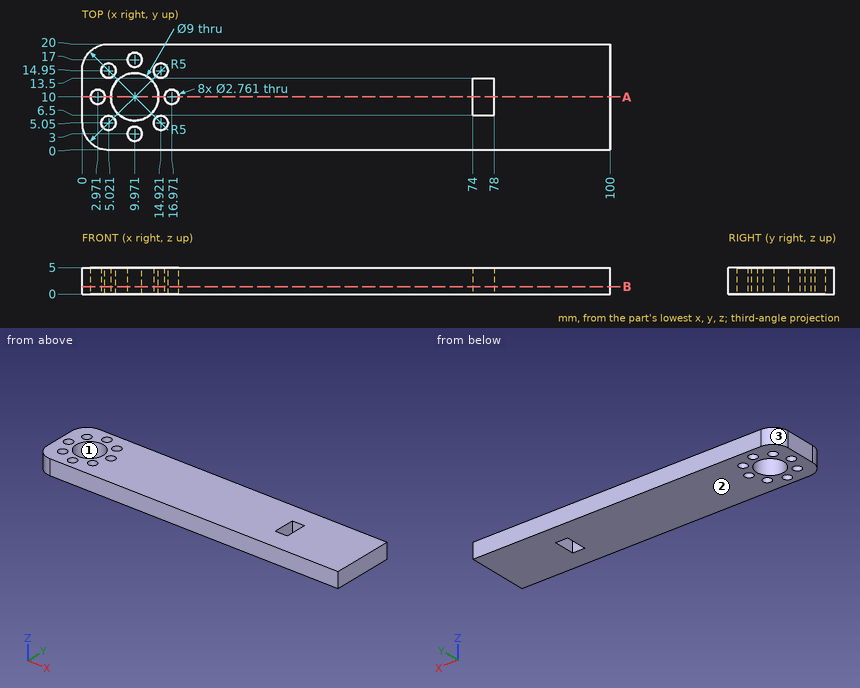
Study the drawing (mm; zero at the part's minimum x, y, z) and answer. Round coordinates to 2 decimals unless told otherwise and drop trailing zeros. Loops run counter-clockwise (first coordinate to the right, second up) from the corner with the lowest first, then second, coordinate; pieces in that order, holes last. Notation, with made-up numbers: (82, 11) -> (123, 11) arc R14 cw to (123, 22) -> close; hole circle Ø10 at (25.5, -34.75). An arc over 180 degrees is marked (long way). Write each question's results on one line, items separated by ' | '. Start each with the question number.
1. Section B-B (z = 1.4) is taken. State how many separate pieces and enclosed holes the cut face has, plus the area to 3 significant figures.
2. For a pull along X with two mould halves and no side action, classify the marked faces 1, 2 and 3 as +X half, -X half, draft (parallel to the pull), parting line (faces both ways), or undercut.
3. Section A-A (y = 10) is taken. Determine the outline of the cut face in (x, z).
4. Find the intervals of material crossed by probe 1 along X at (y, z) = (5.25, 4.45) (1 decimal); probe 2 along X at (y, z) = (10, 2.2); probe 3 along Y at (x, z) = (75.5, 3.35), in increasing order. Write a range as from..to.
Evaluation:
1) separate pieces: 1 | enclosed holes: 10 | area: 1,850 mm2
2) face 1: undercut | face 2: draft | face 3: -X half
3) outline: (0, 0) -> (1.59, 0) -> (1.59, 5) -> (0, 5) -> close; (4.35, 0) -> (5.47, 0) -> (5.47, 5) -> (4.35, 5) -> close; (14.47, 0) -> (15.59, 0) -> (15.59, 5) -> (14.47, 5) -> close; (18.35, 0) -> (74, 0) -> (74, 5) -> (18.35, 5) -> close; (78, 0) -> (100, 0) -> (100, 5) -> (78, 5) -> close
4) probe 1: x = 0..3.7, 6.4..13.6, 16.3..100 | probe 2: x = 0..1.59, 4.35..5.47, 14.47..15.59, 18.35..74, 78..100 | probe 3: y = 0..6.5, 13.5..20
